The listing builds one solid part. Answer for the finished solid, in the listing's coordinates (mm). A direction names the side the tool comes from. Round coordinates to 2 decimals unless told otherwise and drop trailing zeros. Write each loop counter-clockwise with the first axis right and the second up, starting at its lowest first coordinate (ties: lowest second). Pieces come first, ordered by that corner, then holes. Notation, with made-up numbers: M 75,73 L 95,73 A18 cw 95,83 Z; hole C 53,-36.75 d4. An arc over 180 degrees is marked long. Write each question's results on one line, items separated by ' | '.
from build123d import *

# Parameters (mm, degrees)
LOFT1_DEPTH             = 30
LOFT1_DRAFT             = 1.9091524
CUT_EXTRUDE2_DEPTH      = 32.988279093
CUT_EXTRUDE2_DEPTH_BACK = 32.988279093
FILLET2_R               = 1
SKETCH4_R               = 3
BOSS_EXTRUDE1_DEPTH     = 1.5
CUT_EXTRUDE3_START      = 3
SKETCH5_R               = 3
CUT_EXTRUDE3_DEPTH      = 3
SKETCH6_R               = 3
CUT_EXTRUDE4_DEPTH      = 1.5
BOSS_EXTRUDE2_START     = -3
SKETCH7_R               = 3
BOSS_EXTRUDE2_DEPTH     = 3
CUT_EXTRUDE5_DEPTH      = 22.529931357
CUT_EXTRUDE5_DEPTH_BACK = 22.529931357
CUT_EXTRUDE6_DEPTH      = 22.746838212
CUT_EXTRUDE6_DEPTH_BACK = 22.746838212
CUT_EXTRUDE7_DEPTH      = 36.188368954
CUT_EXTRUDE7_DEPTH_BACK = 36.188368954
SKETCH10_R              = 1.45


# Read off the part's stored shape, not the designer's step: Loft1
with BuildPart() as part:
    # Loft1 outline → Loft1 (with draft: the straight prism first)
    with BuildSketch(Plane(origin=(0, 30, 0), x_dir=(1, 0, 0), z_dir=(0, 1, 0))):
        Polygon((2.085786438, 5.5), (-2.085786438, 5.5), (-7.585786438, 0), (-2.085786438, -5.5), (2.085786438, -5.5), (7.585786438, 0), align=None)
    extrude(amount=-LOFT1_DEPTH)
    # Loft1: the draft: its side faces are tilted about the plane it starts from
    loft1_sides = [part.faces().sort_by_distance(p)[0] for p in [
        (0, 15, -5.5),
        (-4.835786438, 15, -2.75),
        (-4.835786438, 15, 2.75),
        (0, 15, 5.5),
        (4.835786438, 15, 2.75),
        (4.835786438, 15, -2.75),
    ]]
    draft(loft1_sides, Plane(origin=(0, 30, 0), x_dir=(1, 0, 0), z_dir=(0, 1, 0)), LOFT1_DRAFT)

    # Sketch3 → Cut-Extrude2 (cut, two sides: drawn at the far end of the back side and taken through both)
    with BuildSketch(Plane(origin=(0, 0, 0), x_dir=(0, 0, -1), z_dir=(1, 0, 0)).offset(-CUT_EXTRUDE2_DEPTH_BACK)):
        Polygon((0, 30), (0, 29), (-5.724137931, 23.275862069), (-5.5, 30), align=None)
        Polygon((0, 0), (0, 1), (-6.258064516, 7.258064516), (-6.5, 0), align=None)
    extrude(amount=CUT_EXTRUDE2_DEPTH + CUT_EXTRUDE2_DEPTH_BACK, mode=Mode.SUBTRACT)

    # Fillet2
    # the kernel refuses this fillet: 1 mm, written as the material it takes off along each edge
    with BuildSketch(Plane(origin=(-7.515337072, 31.494456763, 0), x_dir=(0.70593033942015, -0.0332778747610444, -0.7074990734534851), z_dir=(-0.04708816012216718, -0.9988907373563483, 0))) as fillet2_piece_1:
        with BuildLine():
            CenterArc((FILLET2_R * 0.998890737356, FILLET2_R), FILLET2_R, 180.063591331, 89.936408669)
            Line((-FILLET2_R * 0.00110864672901, FILLET2_R * 0.998890122125), (0, 0))
            Line((0, 0), (FILLET2_R * 0.998890737356, 0))
        make_face()
    extrude(amount=33.025547532, mode=Mode.SUBTRACT)
    with BuildSketch(Plane(origin=(7.515337072, 31.494456763, 0), x_dir=(-0.7059303394201507, -0.03327787476104443, -0.7074990734534845), z_dir=(0.04708816012216718, -0.9988907373563483, 0))) as fillet2_piece_2:
        with BuildLine():
            CenterArc((FILLET2_R * 0.998890737356, -FILLET2_R), FILLET2_R, 90, 89.936408669)
            Line((-FILLET2_R * 0.00110864672901, -FILLET2_R * 0.998890122125), (0, 0))
            Line((0, 0), (FILLET2_R * 0.998890737356, 0))
        make_face()
    extrude(amount=33.025547532, mode=Mode.SUBTRACT)

    # Sketch4 → Boss-Extrude1 (add, symmetric)
    with BuildSketch(Plane(origin=(0, 0, 0), x_dir=(0, 0, -1), z_dir=(1, 0, 0))):
        with Locations((0, 30.5)):
            Circle(SKETCH4_R)
    extrude(amount=BOSS_EXTRUDE1_DEPTH, both=True)

    # Sketch5 → Cut-Extrude3 (cut)
    with BuildSketch(Plane(origin=(1.5, 0, 0), x_dir=(0, 0, -1), z_dir=(1, 0, 0)).offset(CUT_EXTRUDE3_START)):
        with Locations((0, 30.5)):
            Circle(SKETCH5_R)
    cut_extrude3 = extrude(amount=-CUT_EXTRUDE3_DEPTH, mode=Mode.SUBTRACT)

    # Mirror1: Cut-Extrude3 across plane
    add(cut_extrude3.mirror(Plane(origin=(0, 0, 0), x_dir=(0, 0, 1), z_dir=(1, 0, 0))), mode=Mode.SUBTRACT)

    # Sketch6 → Cut-Extrude4 (cut, symmetric)
    with BuildSketch(Plane(origin=(0, 0, 0), x_dir=(0, 0, -1), z_dir=(1, 0, 0))):
        with Locations((0, -0.5)):
            Circle(SKETCH6_R)
    extrude(amount=CUT_EXTRUDE4_DEPTH, both=True, mode=Mode.SUBTRACT)

    # Sketch7 → Boss-Extrude2 (add)
    with BuildSketch(Plane.ZY.offset(-1.5).offset(BOSS_EXTRUDE2_START)):
        with Locations((0, -0.5)):
            Circle(SKETCH7_R)
    boss_extrude2 = extrude(amount=BOSS_EXTRUDE2_DEPTH)

    # Mirror2: Boss-Extrude2 across plane
    add(boss_extrude2.mirror(Plane(origin=(0, 0, 0), x_dir=(0, 0, 1), z_dir=(1, 0, 0))))

    # Sketch8 → Cut-Extrude5 (cut, two sides: drawn at the far end of the back side and taken through both)
    with BuildSketch(Plane(origin=(0, 15.050537099, -0.50168457), x_dir=(1, 0, 0), z_dir=(0, 0.9994449069791544, -0.0333148302326385)).offset(-CUT_EXTRUDE5_DEPTH_BACK)):
        Polygon((-0.75, -4.246391895), (0.75, -4.246391895), (0.75, -4.996391895), (0, -5.746391895), (-0.75, -4.996391895), align=None)
    extrude(amount=CUT_EXTRUDE5_DEPTH + CUT_EXTRUDE5_DEPTH_BACK, mode=Mode.SUBTRACT)

    # Sketch9 → Cut-Extrude6 (cut, two sides: drawn at the far end of the back side and taken through both)
    with BuildSketch(Plane(origin=(0, 14.783573807, 0.492785794), x_dir=(1, 0, 0), z_dir=(0, 0.9994449069791544, 0.0333148302326385)).offset(-CUT_EXTRUDE6_DEPTH_BACK)):
        Polygon((-0.75, 5.746391895), (0.75, 5.746391895), (0.75, 4.996391895), (0, 4.246391895), (-0.75, 4.996391895), align=None)
    extrude(amount=CUT_EXTRUDE6_DEPTH + CUT_EXTRUDE6_DEPTH_BACK, mode=Mode.SUBTRACT)

    # Sketch10 → Cut-Extrude7 (cut, two sides: drawn at the far end of the back side and taken through both)
    with BuildSketch(Plane(origin=(0, 0, 0), x_dir=(0, 0, -1), z_dir=(1, 0, 0)).offset(-CUT_EXTRUDE7_DEPTH_BACK)):
        with Locations((0, 30.5)):
            Circle(SKETCH10_R)
        with Locations((0, -0.5)):
            Circle(SKETCH10_R)
    extrude(amount=CUT_EXTRUDE7_DEPTH + CUT_EXTRUDE7_DEPTH_BACK, mode=Mode.SUBTRACT)


solid = part.part
1) Each of these flat-tipped pins is pushed along its axis until it touches: pin 1 (8 mm diameter, centred on x = -1, y = 28.5, fed in from -Z); pin 2 (3 mm diameter, centred on x = 6.5, y = 19.5, fed in from +Z); pin 3 (1.5 mm diameter, centred on x = -1, y = 27.5, fed in from -Z); pin 4 (2.5 mm diameter, centred on y = -0.5, z = 0, fed in from +X). Where does it stop, or does it pass through?
Return value:
pin 1: z = -5.68 | pin 2: z = 3.08 | pin 3: z = -5.61 | pin 4: through
2) The mould has two halves that part along X. Classify faces 1 (the face through (0, 26, 3)), 2 (the face through (7.87, 15.21, -0.01)), 3 (the face through (0.75, 15, 4)), 4 (the face through (-1.5, 29, 1)): +X half, -X half, draft (parallel to the pull), parting line (faces both ways), or undercut.
Return value:
face 1: draft | face 2: +X half | face 3: undercut | face 4: undercut
3) Section A-A (y = 30.5) is taken. Determine the outline of the cut face in (x, z).
Return value:
outline: M -1.5,-3 L 1.5,-3 L 1.5,-1.45 L -1.5,-1.45 Z; M -1.5,1.45 L 1.5,1.45 L 1.5,3 L -1.5,3 Z
4) A tool of negligible diameter and unlimited length cuts with its end or side. For faces 5 (the face through (-4.5, -2, 1)), 6 (the face through (3.021, 27.835, -1.377)), 7 (the face through (-0.75, 15, 4)), from which of +Z, -Z, +X, -X, +Y, -Y can it reach the whole face along a straight path? Write none if from no direction.
Return value:
face 5: +Z, -X, -Y | face 6: +Y | face 7: none
5) Section C-C (x = 3) is taken. Determine the outline of the cut face in (y, z).
Return value:
outline: M 0,-6 L 30,-4.59 L 30,-2.96 A3 cw 27.77,1.23 L 24.14,4.86 L 6.68,5.68 L 2.23,1.23 A3 ccw long 0,-2.96 Z; hole C -0.5,0 d2.9
6) Section D-D (x = 5) is taken. Determine the outline of the cut face in (y, z), then the cut area to 3 significant figures.
Return value:
outline: M 0,-4 L 30,-2.59 L 30,-1.36 A1.45 cw 29.05,0 L 29,0 L 26.24,2.76 L 4.77,3.77 L 1,0 L 0.95,0 A1.45 cw 0,-1.36 Z | area: 178 mm²
7) Section B-B (y = -0.5) is taken. Determine the outline of the cut face in (x, z).
Return value:
outline: M -4.5,-3 L -1.5,-3 L -1.5,-1.45 L -4.5,-1.45 Z; M -4.5,1.45 L -1.5,1.45 L -1.5,3 L -4.5,3 Z; M 1.5,-3 L 4.5,-3 L 4.5,-1.45 L 1.5,-1.45 Z; M 1.5,1.45 L 4.5,1.45 L 4.5,3 L 1.5,3 Z
8) Find the intervals of material crossed by line 1 (Z direction, x = -0.75, y = 30.5); line 2 (Z direction, x = -0.5, y = 22); line 3 (Y direction, x = -0.55, z = 0), in increasing order.
Return value:
line 1: -3 to -1.45, 1.45 to 3 | line 2: -5.77 to -5.02, -4.02 to 3.52, 4.52 to 5.77 | line 3: 2.5 to 29.05, 31.95 to 33.5
